Design review of the part shown in the three views and the two pictorial views. Dimensions are in mm from the part's minimum x, y and z. A direction names the side the tool comes from. Coordinates: 2 decimals unless noted, no trailing zeros. Write each loop counter-clockwise with the first axis right and the second up, starting at its lowest first coordinate (ties: lowest second). Pieces come first, ordered by that corner, then holes. Notation, with made-up numbers: (9.25, 64) -> (45.25, 64) arc R24 cw to (45.25, 80) -> close; hole circle Ø5 at (56, 46). An arc over 180 degrees is marked (long way). Write item = value, one per line. Start each with the question number.
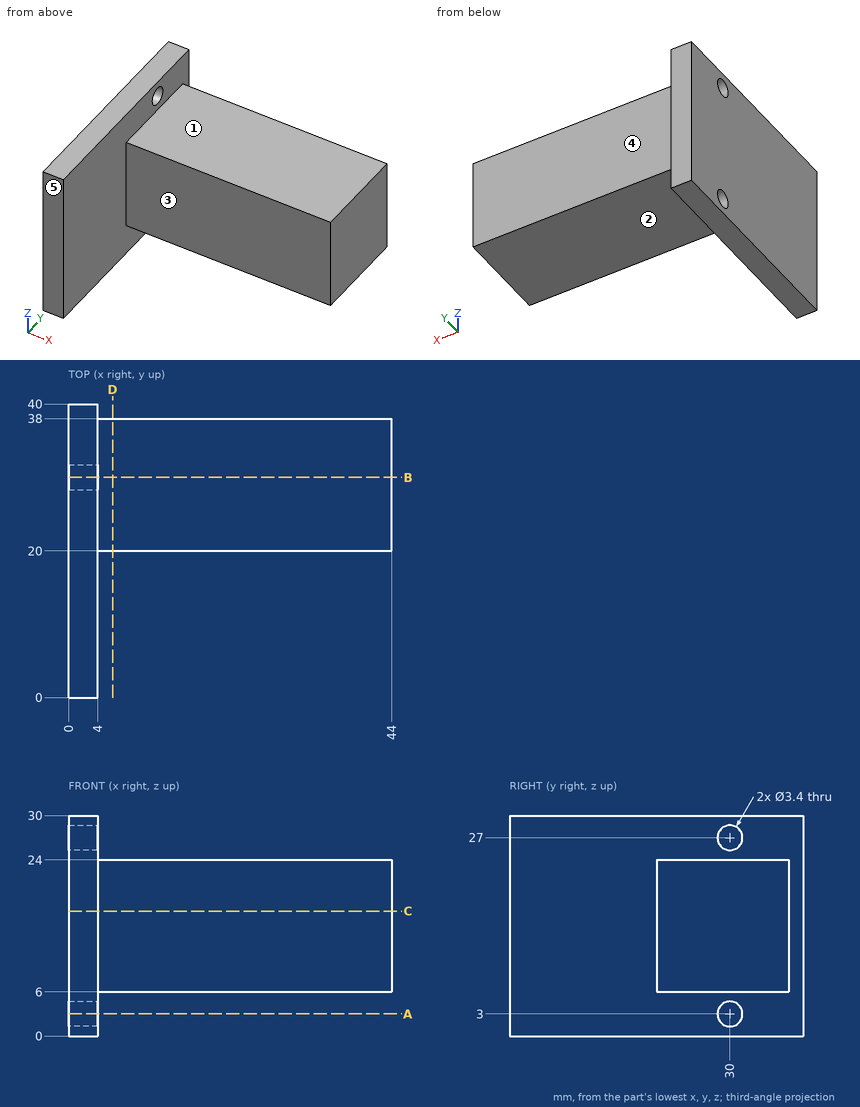
(1) For the marked faces 1, 2, 3, 4 and 5, list the 3-axis set-ups (+Z, -Z, +X, -X, +Y, -Y) from which the entire face can be reached by the end or side of a thin tool; tool diameter is ignored.
(2) For line 1 (Y direction, x = 3, z = 27); line 2 (Y direction, x = 22, z = 9.75); line 3 (X direction, y = 9.5, z = 2), list the stretches that pass through material, from the lowest coordinate up.
(3) Take a section at A-A, the plane z = 3. State the section outline as (x, y) points.
(4) For pin 1 Ø14.5 at (x, z) = (15, 11) entering from +Y; pin 2 Ø6 at (x, y) = (37, 31) entering from -Z; pin 3 Ø20 at (x, y) = (21.5, 27.5) entering from +Z, all flat-tipped, find the tip position at first contact; note any pin that passes through.
(5) Take a section at D-D, the plane x = 6. State the section outline as (y, z) points, then the cut area to 3 significant figures.
(6) Take a section at B-B, the plane y = 30. State the section outline as (x, z) points, then the cut area to 3 significant figures.
(7) Take a section at C-C, the plane z = 17. State the section outline as (x, y) points.
Report:
q1.face_1 = +Z, +X, +Y, -Y
q1.face_2 = -Z, +X, +Y, -Y
q1.face_3 = +Z, -Z, +X, -Y
q1.face_4 = +Z, -Z, +X, +Y
q1.face_5 = +Z, -Z, +X, -X, -Y
q2.line_1 = 0 to 28.3, 31.7 to 40
q2.line_2 = 20 to 38
q2.line_3 = 0 to 4
q3.outline = (0, 0) -> (4, 0) -> (4, 28.3) -> (0, 28.3) -> close; (0, 31.7) -> (4, 31.7) -> (4, 40) -> (0, 40) -> close
q4.pin_1 = 38
q4.pin_2 = 6
q4.pin_3 = 24
q5.outline = (20, 6) -> (38, 6) -> (38, 24) -> (20, 24) -> close
q5.area = 324 mm2
q6.outline = (0, 0) -> (4, 0) -> (4, 1.3) -> (0, 1.3) -> close; (0, 4.7) -> (4, 4.7) -> (4, 6) -> (44, 6) -> (44, 24) -> (4, 24) -> (4, 25.3) -> (0, 25.3) -> close; (0, 28.7) -> (4, 28.7) -> (4, 30) -> (0, 30) -> close
q6.area = 813 mm2
q7.outline = (0, 0) -> (4, 0) -> (4, 20) -> (44, 20) -> (44, 38) -> (4, 38) -> (4, 40) -> (0, 40) -> close
